Work out the finished part from the listing and answer in its coordinate system (mm). A direction names the side the tool comes from. Round coordinates to 2 decimals unless told otherwise and drop trailing zeros. Write each loop counter-clockwise with the first axis right and the second up, starting at its lowest first coordinate (ties: lowest second). Pieces come first, ordered by that corner, then holes. Notation, with made-up numbers: (83, 8) -> (118, 8) arc R17 ccw to (118, 13) -> close; hole circle Ø7 at (14, -20). An arc over 180 degrees is marked (long way). One line per item, written item: value.
```python
from build123d import *

# Parameters (mm, degrees)
SKETCH1_R           = 1.7
BOSS_EXTRUDE1_DEPTH = 5
CUT_EXTRUDE1_START  = -5
CUT_EXTRUDE1_DEPTH  = 4
BOSS_EXTRUDE2_DEPTH = 6
BOSS_EXTRUDE3_DEPTH = 0.75
BOSS_EXTRUDE4_DEPTH = 7.5
SKETCH7_R           = 1.3
CUT_EXTRUDE2_DEPTH  = 7.5


with BuildPart() as part:
    # Sketch1 → Boss-Extrude1 (new body)
    with BuildSketch(Plane(origin=(0, 0, 0), x_dir=(1, 0, 0), z_dir=(0, 1, 0))):
        with BuildLine():
            Line((-4.494644994, 13.719468408), (-4.772250922, 8.034184997))
            ThreePointArc((-4.772250922, 8.034184997), (-6.10009687, 3.52189257), (-9.343933767, 0.115798034))
            Line((-9.343933767, 0.115798034), (-14.128730664, -2.967257459))
            ThreePointArc((-14.128730664, -2.967257459), (-15.588457268, -9), (-9.634085671, -10.752210949))
            Line((-9.634085671, -10.752210949), (-4.571682845, -8.149983031))
            ThreePointArc((-4.571682845, -8.149983031), (0, -7.04378514), (4.571682845, -8.149983031))
            Line((4.571682845, -8.149983031), (9.634085671, -10.752210949))
            ThreePointArc((9.634085671, -10.752210949), (15.588457268, -9), (14.128730664, -2.967257459))
            Line((14.128730664, -2.967257459), (9.343933767, 0.115798034))
            ThreePointArc((9.343933767, 0.115798034), (6.10009687, 3.52189257), (4.772250922, 8.034184997))
            Line((4.772250922, 8.034184997), (4.494644994, 13.719468408))
            ThreePointArc((4.494644994, 13.719468408), (0, 18), (-4.494644994, 13.719468408))
        make_face()
        with Locations((0, 13.5)):
            Circle(SKETCH1_R, mode=Mode.SUBTRACT)
        with Locations((11.691342951, -6.75)):
            Circle(SKETCH1_R, mode=Mode.SUBTRACT)
        with Locations((-11.691342951, -6.75)):
            Circle(SKETCH1_R, mode=Mode.SUBTRACT)
    extrude(amount=BOSS_EXTRUDE1_DEPTH)

    # Sketch2 → Cut-Extrude1 (cut)
    with BuildSketch(Plane(origin=(0, 5, 0), x_dir=(1, 0, 0), z_dir=(0, 1, 0)).offset(CUT_EXTRUDE1_START)):
        Polygon((14.441342951, -8.33771324), (14.441342951, -5.16228676), (11.691342951, -3.574573519), (8.941342951, -5.16228676), (8.941342951, -8.33771324), (11.691342951, -9.925426481), align=None)
        Polygon((0, 16.675426481), (-2.75, 15.08771324), (-2.75, 11.91228676), (0, 10.324573519), (2.75, 11.91228676), (2.75, 15.08771324), align=None)
        Polygon((-14.441342951, -8.33771324), (-11.691342951, -9.925426481), (-8.941342951, -8.33771324), (-8.941342951, -5.16228676), (-11.691342951, -3.574573519), (-14.441342951, -5.16228676), align=None)
    extrude(amount=CUT_EXTRUDE1_DEPTH, mode=Mode.SUBTRACT)

    # Sketch4 → Boss-Extrude2 (add)
    with BuildSketch(Plane.XZ):
        with BuildLine():
            ThreePointArc((-4.872953171, -7.025441438), (0, -8.55), (4.872953171, -7.025441438))
            ThreePointArc((4.872953171, -7.025441438), (6.10009687, -3.52189257), (8.520687343, -0.707380519))
            ThreePointArc((8.520687343, -0.707380519), (7.404517202, 4.275), (3.647734172, 7.732821956))
            ThreePointArc((3.647734172, 7.732821956), (0, 7.04378514), (-3.647734172, 7.732821956))
            ThreePointArc((-3.647734172, 7.732821956), (-7.404517202, 4.275), (-8.520687343, -0.707380519))
            ThreePointArc((-8.520687343, -0.707380519), (-6.10009687, -3.52189257), (-4.872953171, -7.025441438))
        make_face()
    extrude(amount=BOSS_EXTRUDE2_DEPTH)

    # Sketch5 → Boss-Extrude3 (add)
    with BuildSketch(Plane.XZ):
        with BuildLine():
            Line((-9.499987767, -0.015245565), (-8.520687343, -0.707380519))
            ThreePointArc((-8.520687343, -0.707380519), (-7.404517202, 4.275), (-3.647734172, 7.732821956))
            Line((-3.647734172, 7.732821956), (-4.736790837, 8.234853524))
            ThreePointArc((-4.736790837, 8.234853524), (-8.227241336, 4.75), (-9.499987767, -0.015245565))
        make_face()
        with BuildLine():
            Line((9.499987767, -0.015245565), (8.520687343, -0.707380519))
            ThreePointArc((8.520687343, -0.707380519), (7.404517202, 4.275), (3.647734172, 7.732821956))
            Line((3.647734172, 7.732821956), (4.736790837, 8.234853524))
            ThreePointArc((4.736790837, 8.234853524), (8.227241336, 4.75), (9.499987767, -0.015245565))
        make_face()
        with BuildLine():
            Line((-4.76319693, -8.219607959), (-4.872953171, -7.025441438))
            ThreePointArc((-4.872953171, -7.025441438), (0, -8.55), (4.872953171, -7.025441438))
            Line((4.872953171, -7.025441438), (4.76319693, -8.219607959))
            ThreePointArc((4.76319693, -8.219607959), (0, -9.5), (-4.76319693, -8.219607959))
        make_face()
    extrude(amount=BOSS_EXTRUDE3_DEPTH)

    # Sketch6 → Boss-Extrude4 (add)
    with BuildSketch(Plane.XZ.offset(6)):
        with BuildLine():
            Line((-0.75, 2.90473751), (-0.75, 3.90473751))
            Line((-0.75, 3.90473751), (0.75, 3.90473751))
            Line((0.75, 3.90473751), (0.75, 2.90473751))
            ThreePointArc((0.75, 2.90473751), (0, -3), (-0.75, 2.90473751))
        make_face()
    extrude(amount=BOSS_EXTRUDE4_DEPTH)

    # Sketch7 → Cut-Extrude2 (cut)
    with BuildSketch(Plane.XZ.offset(13.5)):
        Circle(SKETCH7_R)
    extrude(amount=-CUT_EXTRUDE2_DEPTH, mode=Mode.SUBTRACT)


solid = part.part
```
(1) Find section A-A on y = -3. Give the vertices of the cut face in (x, z).
Reported:
outline: (-8.52, -0.71) arc R10 cw to (-4.87, -7.03) arc R8.55 ccw to (4.87, -7.03) arc R10 cw to (8.52, -0.71) arc R8.55 ccw to (3.65, 7.73) arc R10 cw to (-3.65, 7.73) arc R8.55 ccw to start
(2) For a pull along Z with two mould halves and no side action, classify faces 4 (the face through (1.36, 1.97, -11.11)), 5 (the face through (-1.3, 4, -12.1)), 6 (the face through (8.7, 0, 6.8)), 7 (the face through (0, -10, -3)) as pulls with the +Z half, pulls with the -Z half, needs draft (parallel to the pull), parting line crosses it, or undercut.
Reported:
face 4: undercut
face 5: undercut
face 6: needs draft
face 7: parting line crosses it
(3) Flat-ended cylindrical pins translate along their axes: pin 1 Ø0.5 at (y, z) = (-11, 3) entering from +X; pin 2 Ø3 at (x, z) = (-10.5, 5.5) entering from -Y; pin 3 Ø1.6 at (y, z) = (2, -14) entering from +X. Find the tip coordinate at first contact, or state that the pin passes through.
Reported:
pin 1: stops at x = 1.2
pin 2: stops at y = 0
pin 3: stops at x = 4.52
(4) Find section D-D on x = -6. Give the vertices of the cut face in (y, z).
Reported:
outline: (-6, -3.7) -> (5, -3.7) -> (5, 8.88) -> (0, 8.88) -> (0, 7.37) -> (-0.75, 7.37) -> (-0.75, 6.09) -> (-6, 6.09) -> close
(5) Find section C-C on z = -11.25. Give the vertices of the cut face in (x, y).
Reported:
outline: (-4.62, 0) -> (-1.6, 0) -> (-1.6, 4) -> (1.6, 4) -> (1.6, 0) -> (4.62, 0) -> (4.62, 5) -> (-4.62, 5) -> close
(6) A tool of negligible diameter and unlimited length cuts with its end or side. For faces 1 (the face through (-7.14, 2.46, 9.47)), 2 (the face through (13.09, 1.97, 4.38)), 3 (the face through (12.476, 4.493, 8.258)), from which of +Z, -Z, +X, -X, +Y, -Y can it reach the whole face along a straight path? Write none if from no direction.
Reported:
face 1: +Z, +Y, -Y
face 2: -Y
face 3: +Y, -Y
(7) Consider probe 1 along X at (y, z) = (4.8, 6.75); probe 2 along X at (y, z) = (2, 5.25); probe 3 along Y at (x, z) = (5, -4.5). Determine where each line is inside the solid, lowest interval first.
Reported:
probe 1: x = -16.19 to -13.39, -9.99 to 9.99, 13.39 to 16.19
probe 2: x = -15.93 to -14.44, -8.94 to 8.94, 14.44 to 15.93
probe 3: y = -6 to 5
(8) Find section B-B on y = -7.5. Give the vertices of the cut face in (x, z).
Reported:
outline: (-0.75, 2.9) arc R3 ccw (long way) to (0.75, 2.9) -> (0.75, 3.9) -> (-0.75, 3.9) -> close; hole circle Ø2.6 at (0, 0)
